Autodesk Inventor part; units mm, degrees
ref_plane "YZ Plane" through (0, 0, 0) normal (1, 0, 0) x (0, 1, 0)
ref_plane "XZ Plane" through (0, 0, 0) normal (0, 1, 0) x (-1, 0, 0)
ref_plane "XY Plane" through (0, 0, 0) normal (0, 0, 1) x (1, 0, 0)
sketch "Szkic1" plane through (0, 0, 0) normal (0, 0, 1) x (1, 0, 0)
  circle A0 centre (0, 0) radius 10
  circle A1 centre (0, 0) radius 13
  circle A2 centre (0, 0) radius 2.45
  line L0 (0, -13) -> (32, -13)
  line L1 (32, -13) -> (32, 13)
  line L2 (32, 13) -> (0, 13)
  line L3 (-32, -13) -> (32, 13) construction
  line L4 (32, -13) -> (-32, 13) construction
  dimension "d0" = 20
  dimension "d1" = 26
  dimension "d2" = 4.9
extrude "Wyciągnięcie proste1" add sketch "Szkic1" against normal blind 8 contours A0
extrude "Wyciągnięcie proste2" add sketch "Szkic1" along normal blind 12 contours A0 | A1 | A1 L2 L1 L0 | A2
extrude "Wyciągnięcie proste3" add sketch "Szkic1" against normal blind 20 contours A1 L2 L1 L0
fillet "Zaokrąglenie1" radius 10 6 edges at (16, -13, -20) (-13, 0, 12) (16, 13, 12) (16, -13, 12) (16, 13, -20) (32, 0, 12)
properties part number "cchwytak holdeer"
Here's how the part is built. I have some questions about the finished solid (model axes, mm). A direction names the side the tool comes from. Coordinates: 2 decimals unless noted, no trailing zeros. Order: outer loops, then holes, each group sorted by start corner. A loop starts at its lowest first (then second) coordinate and runs counter-clockwise, first axis right, second up. Notation, with made-up numbers: (38.5, 85) -> (58.5, 85) arc R23 ccw to (58.5, 108) -> close; hole circle Ø10 at (44, 6). An arc over 180 degrees is marked (long way). Answer in a Markdown table with one row per item.
(1) Thinking about a two-plate mould opening in Y: for faces 1 (the face through (-0.5, -2.4, -3.9)), 2 (the face through (13, 0, -8)), 3 (the face through (-13, 0, 1)), 4 (the face through (19.78, -10.15, -16.99)), which applies, +Y half, -Y half, draft (parallel to the pull), parting line (faces both ways), or undercut?
Answer key:
| item | result |
|---|---|
| face 1 | undercut |
| face 2 | undercut |
| face 3 | parting line |
| face 4 | -Y half |
(2) I want a section at A-A on z = -2.5. List the corners of the cut face in (x, y) for me, then the cut area to 3 significant figures.
Answer key:
| item | result |
|---|---|
| outline | circle Ø20 at (0, 0); (0, -13) -> (32, -13) -> (32, 13) -> (0, 13) arc R13 cw to start; hole circle Ø4.9 at (0, 0) |
| area | 862 mm^2 |
(3) On a 3-axis mill with a long thin cutter (end or side, diameter ignored), from which of +Z, -Z, +X, -X, +Y, -Y can I reach the whole of each face in a straight line? I mean faces 5 (the face through (9, 0, 12)), 6 (the face through (-2.17, -9.76, -3.94)), 7 (the face through (2, -2, -8)). Say none if no direction works.
Answer key:
| item | result |
|---|---|
| face 5 | +Z, +X, -X, +Y, -Y |
| face 6 | -Z |
| face 7 | -Z, -X |
(4) Please list where these lines run through material, in increasing order: probe 1 along X at (y, z) = (-0.75, -6.5); probe 2 along X at (y, z) = (5, -17); probe 3 along Y at (x, z) = (-8.5, 1).
Answer key:
| item | result |
|---|---|
| probe 1 | -9.97 to -2.33, 2.33 to 9.97, 12.98 to 32 |
| probe 2 | 12 to 32 |
| probe 3 | -9.84 to 9.84 |
(5) Will these pins go through, and if not, where does the flat tip stop? pin 1 Ø6 at (x, y) = (22, -5) entering from -Z; pin 2 Ø5 at (x, z) = (9.5, -15.5) entering from -Y; pin 3 Ø4 at (x, z) = (9, -15.5) entering from -Y; pin 4 Ø8 at (x, z) = (-3.5, 4.5) entering from +Y.
Answer key:
| item | result |
|---|---|
| pin 1 | z = -20 |
| pin 2 | y = -12.54 |
| pin 3 | y = -12.37 |
| pin 4 | y = 13 |
(6) I want a section at B-B on z = -12.5. List the corners of the cut face in (x, y) for me, then the cut area to 3 significant figures.
Answer key:
| item | result |
|---|---|
| outline | (2.86, -12.68) -> (32, -12.68) -> (32, 12.68) -> (2.86, 12.68) arc R13 cw to start |
| area | 547 mm^2 |
